```python
from build123d import *

# Parameters (mm, degrees)
F0_R          = 9
F1_DEPTH      = 10
F1_DEPTH_BACK = 1.5
F2_W          = 51.6399771267
F2_H          = 119.0588462234
F2_R          = 11
F3_DEPTH      = 6.35
F4_W          = 51.6399771267
F4_H          = 119.0588462234
F5_DEPTH      = 6.35


with BuildPart() as f1:
    # F0 (on Front) → F1 (new body, two sides)
    with BuildSketch(Plane.XZ) as f1_sk:
        Circle(F0_R)
    extrude(amount=-F1_DEPTH)
    extrude(f1_sk.sketch, amount=F1_DEPTH_BACK)



with BuildPart() as f3:
    # F2 (on Front) → F3 (new body)
    with BuildSketch(Plane.XZ):
        Rectangle(F2_W, F2_H)
        Circle(F2_R, mode=Mode.SUBTRACT)
    extrude(amount=-F3_DEPTH)


with BuildPart() as f1_1:
    add(f1.part)

    add(f3.part)  # F5 merges F3
    # F4 (on face) → F5 (join)
    with BuildSketch(Plane(origin=(0, 6.35, 0), x_dir=(-1, 0, 0), z_dir=(0, 1, 0))):
        Rectangle(F4_W, F4_H)
    extrude(amount=F5_DEPTH)


solid = f1_1.part
```
Model file for the job. Use its own axes, mm. A direction names the side the tool comes from. Coordinates: 2 decimals unless noted, no trailing zeros. Write each loop counter-clockwise with the first axis right and the second up, starting at its lowest first coordinate (ties: lowest second). Pieces come first, ordered by that corner, then holes. Notation, with made-up numbers: (85.5, 58) - (89.5, 58) arc R8 cw to (89.5, 64) - close; hole circle Ø1 at (73.5, 12.5). An arc over 180 degrees is marked (long way). One line per question, with ' | ' between items. Start each with the question number.
Q1. Cut at C-C, the plane z = 0. List the corners of the cut face in (x, y), then the cut area to 3 significant figures.
Q2. 3-axis set-ups, long thin cutter, end or side, ignore diameter. For faces 4 (the face through (-2.38, 3.13, -10.74)), 5 (the face through (0, -1.5, 0)): which of +Z, -Z, +X, -X, +Y, -Y reach the whole face in a straight line?
Q3. Pull direction Z, two halves, no side cores. Call faces 1 (the face through (0, 6, -59.529)), 2 (the face through (25.82, 6, -1)), 3 (the face through (-2, 6.35, -9)): pulls with the +Z half, pulls with the -Z half, needs draft (parallel to the pull), parting line crosses it, or undercut.
Q4. Cut at D-D, the plane z = -27.5. List the corners of the cut face in (x, y), then the cut area to 3 significant figures.
Q5. Drill centre lines: line 1 (Z direction, x = 0, y = 5.25); line 2 (Z direction, x = 5, y = 4.25); line 3 (Y direction, x = 13, z = -41). Where is each one in solid material? Low to high. Write a range as [from, to].
Q6. Cut at B-B, the plane x = 0. List the corners of the cut face in (y, z), then the cut area to 3 significant figures.
Q7. Cut at A-A, the plane y = 5.25. List the corners of the cut face in (x, z), then the cut area to 3 significant figures.
Answer below:
1) outline: (-25.82, 0) - (-11, 0) - (-11, 6.35) - (-9, 6.35) - (-9, -1.5) - (9, -1.5) - (9, 6.35) - (11, 6.35) - (11, 0) - (25.82, 0) - (25.82, 12.7) - (-25.82, 12.7) - close | area: 657 mm^2
2) face 4: -Y | face 5: +Z, -Z, +X, -X, -Y
3) face 1: pulls with the -Z half | face 2: needs draft | face 3: undercut
4) outline: (-25.82, 0) - (25.82, 0) - (25.82, 12.7) - (-25.82, 12.7) - close | area: 656 mm^2
5) line 1: [-59.53, -11], [-9, 9], [11, 59.53] | line 2: [-59.53, -9.8], [-7.48, 7.48], [9.8, 59.53] | line 3: [0, 12.7]
6) outline: (-1.5, -9) - (6.35, -9) - (6.35, -11) - (0, -11) - (0, -59.53) - (12.7, -59.53) - (12.7, 59.53) - (0, 59.53) - (0, 11) - (6.35, 11) - (6.35, 9) - (-1.5, 9) - close | area: 1,510 mm^2
7) outline: (-25.82, -59.53) - (25.82, -59.53) - (25.82, 59.53) - (-25.82, 59.53) - close; circle Ø18 at (0, 0); hole circle Ø22 at (0, 0) | area: 6,020 mm^2
